```python
from build123d import *
from OCP.BRepFilletAPI import BRepFilletAPI_MakeChamfer

# Parameters (mm, degrees)
SKETCH1_W                = 40
SKETCH1_H                = 48
BOSS_EXTRUDE1_DEPTH      = 4
BOSS_EXTRUDE2_DEPTH      = 11.15
BOSS_EXTRUDE2_DEPTH_BACK = 4
SKETCH5_W                = 40
SKETCH5_H                = 4.325
SKETCH5_W_2              = 18
SKETCH5_H_2              = 5
SKETCH5_H_3              = 6
FILLET1_R                = 4
SKETCH6_R                = 1.35
CUT_EXTRUDE4_DEPTH       = 58.214705278
CHAMFER2_SIZE            = 2
SKETCH7_W                = 40
SKETCH7_H                = 6.5
CUT_EXTRUDE5_DEPTH       = 3
FILLET2_R                = 3
CHAMFER3_SIZE            = 3
CHAMFER3_SIZE2           = 1
CHAMFER4_SIZE            = 3
CHAMFER4_SIZE2           = 0.5
CUT_EXTRUDE6_DEPTH       = 10
CUT_EXTRUDE6_DEPTH_BACK  = 10
CUT_EXTRUDE8_REACH       = 66.292
SKETCH12_R               = 3
SKETCH13_R               = 1.5
CUT_EXTRUDE10_DEPTH      = 11.175
CUT_EXTRUDE7_DEPTH       = 1.25
CUT_EXTRUDE7_DEPTH_BACK  = 1.25


with BuildPart() as part:
    # Sketch1 → Boss-Extrude1 (new body)
    with BuildSketch(Plane.XY):
        with Locations((20, 14)):
            Rectangle(SKETCH1_W, SKETCH1_H)
    extrude(amount=BOSS_EXTRUDE1_DEPTH)

    # Sketch5 → Boss-Extrude2 (add, two sides: drawn at the far end of the back side and taken through both)
    with BuildSketch(Plane.XY.offset(4).offset(-BOSS_EXTRUDE2_DEPTH_BACK)):
        Polygon((1.8, 8.125), (0, 8.125), (0, 15.5), (40, 15.5), (40, 8.825), (28, 8.825), (27.1625, 10.5), (13.70350416, 10.5), (12.51600416, 8.125), (10, 8.125), (9.4, 6.925), (7.4, 6.925), (6.8, 8.125), (5, 8.125), (4.4, 6.925), (2.4, 6.925), align=None)
        with Locations((20, 3.1625)):
            Rectangle(SKETCH5_W, SKETCH5_H)
        with Locations((20, -7.5)):
            Rectangle(SKETCH5_W_2, SKETCH5_H_2)
        with Locations((20, 35)):
            Rectangle(SKETCH5_W, SKETCH5_H_3)
    extrude(amount=BOSS_EXTRUDE2_DEPTH + BOSS_EXTRUDE2_DEPTH_BACK)

    # Fillet1
    fillet1_edges = [part.edges().sort_by_distance(p)[0] for p in [
        (20, 32, 4),
        (20, 1, 4),
    ]]
    fillet(fillet1_edges, radius=FILLET1_R)

    # Sketch6 → Cut-Extrude4 (cut, through all)
    with BuildSketch(Plane.XY.offset(15.15)):
        with Locations((7.5, 35)):
            Circle(SKETCH6_R)
        with Locations((7.5, 12)):
            Circle(SKETCH6_R)
        with Locations((32.5, 35)):
            Circle(SKETCH6_R)
        with Locations((32.5, 12)):
            Circle(SKETCH6_R)
    extrude(amount=-CUT_EXTRUDE4_DEPTH, mode=Mode.SUBTRACT)

    # Chamfer2
    chamfer2_edges = [part.edges().sort_by_distance(p)[0] for p in [
        (40, 8.825, 9.575),
        (0, 15.5, 9.575),
        (40, 15.5, 9.575),
    ]]
    chamfer(chamfer2_edges, length=CHAMFER2_SIZE)

    # Sketch7 → Cut-Extrude5 (cut)
    with BuildSketch(Plane.XY.offset(4)):
        with Locations((20, 18.75)):
            Rectangle(SKETCH7_W, SKETCH7_H)
    extrude(amount=-CUT_EXTRUDE5_DEPTH, mode=Mode.SUBTRACT)

    # Fillet2
    fillet2_edges = [part.edges().sort_by_distance(p)[0] for p in [
        (20, 15.5, 1),
        (20, 22, 1),
    ]]
    fillet(fillet2_edges, radius=FILLET2_R - 0.0001)  # a hair under: the kernel refuses the full size

    # Chamfer3: one chamfer whose edges measure the first distance from different faces: ONE call of the kernel's chamfer builder (chamfer() names one face for all edges)
    chamfer3_edges_1 = [part.edges().sort_by_distance(p)[0] for p in [
        (3.4, 6.925, 15.15),
    ]]
    chamfer3_side_1 = [part.faces().sort_by_distance(p)[0] for p in [
        (3.4, 6.925, 9.575),
    ]]
    chamfer3_edges_2 = [part.edges().sort_by_distance(p)[0] for p in [
        (8.4, 6.925, 15.15),
    ]]
    chamfer3_side_2 = [part.faces().sort_by_distance(p)[0] for p in [
        (8.4, 6.925, 9.575),
    ]]
    chamfer3 = BRepFilletAPI_MakeChamfer(part.part.solid().wrapped)
    for e in chamfer3_edges_1:
        chamfer3.Add(CHAMFER3_SIZE, CHAMFER3_SIZE2, e.wrapped, chamfer3_side_1[0].wrapped)  # the first distance lies on this face
    for e in chamfer3_edges_2:
        chamfer3.Add(CHAMFER3_SIZE, CHAMFER3_SIZE2, e.wrapped, chamfer3_side_2[0].wrapped)  # the first distance lies on this face
    add(Compound.cast(chamfer3.Shape()), mode=Mode.REPLACE)

    # Chamfer4
    chamfer4_edges = [part.edges().sort_by_distance(p)[0] for p in [
        (20, 5.325, 15.15),
    ]]
    chamfer4_side = [part.faces().sort_by_distance(p)[0] for p in [
        (20, 5.325, 9.575),
    ]]
    chamfer(chamfer4_edges, length=CHAMFER4_SIZE, length2=CHAMFER4_SIZE2, reference=chamfer4_side[0])

    # Sketch8 → Cut-Extrude6 (cut, two sides: drawn at the far end of the back side and taken through both)
    with BuildSketch(Plane(origin=(20, 0, 0), x_dir=(0, 0, -1), z_dir=(1, 0, 0)).offset(-CUT_EXTRUDE6_DEPTH_BACK)):
        with BuildLine():
            Line((-9, 34.15), (-18.856272107, 34.15))
            Line((-18.856272107, 34.15), (-18.856272107, 21.85))
            Line((-18.856272107, 21.85), (-9, 21.85))
            ThreePointArc((-9, 21.85), (-2.85, 28), (-9, 34.15))
        make_face()
        with BuildLine():
            Line((-18.856272107, -10.437196649), (-18.856272107, -3.158858698))
            Line((-18.856272107, -3.158858698), (-13.348706704, 2.348706704))
            ThreePointArc((-13.348706704, 2.348706704), (-3.318140875, 0.353503109), (-9, -8.15))
            Line((-9, -8.15), (-9, -10.437196649))
            Line((-9, -10.437196649), (-18.856272107, -10.437196649))
        make_face()
    extrude(amount=CUT_EXTRUDE6_DEPTH + CUT_EXTRUDE6_DEPTH_BACK, mode=Mode.SUBTRACT)

    # Cut-Extrude8: up to this face of the body (flat: up to its plane)
    cut_extrude8_end = Plane(part.part.faces().sort_by_distance((20, 15.5, 9.574944444))[0])
    # Sketch12 → Cut-Extrude8 (cut, up to the picked face)
    with BuildSketch(Plane(origin=(0, 38, 0), x_dir=(1, 0, 0), z_dir=(0, 1, 0)), mode=Mode.PRIVATE) as cut_extrude8_sk1:
        with Locations(Location((15.4, -9, 0), (0, 0, 270))):
            Circle(SKETCH12_R)
    cut_extrude8_tool1 = split(extrude(cut_extrude8_sk1.sketch, amount=-CUT_EXTRUDE8_REACH, mode=Mode.PRIVATE), bisect_by=cut_extrude8_end, keep=Keep.BOTH, mode=Mode.PRIVATE)
    add(cut_extrude8_tool1.solids().sort_by(Axis((15.4, 38, 9), (0, -1, 0)))[0], mode=Mode.SUBTRACT)

    # Sketch13 → Cut-Extrude10 (cut)
    with BuildSketch(Plane(origin=(0, 15.5, 0), x_dir=(1, 0, 0), z_dir=(0, 1, 0))):
        with Locations(Location((15.4, -9, 0), (0, 0, 180))):
            Circle(SKETCH13_R)
    extrude(amount=-CUT_EXTRUDE10_DEPTH, mode=Mode.SUBTRACT)

    # Sketch9 → Cut-Extrude7 (cut, two sides: drawn at the far end of the back side and taken through both)
    with BuildSketch(Plane.XZ.offset(-13).offset(-CUT_EXTRUDE7_DEPTH_BACK)):
        Polygon((12.5, 16.815347994), (18.3, 16.815347994), (18.3, 7.325684219), (15.4, 5.651368439), (12.5, 7.325684219), align=None)
    extrude(amount=CUT_EXTRUDE7_DEPTH + CUT_EXTRUDE7_DEPTH_BACK, mode=Mode.SUBTRACT)


solid = part.part
```
Design review of the part built by this model. Coordinates are the model's own, in mm. A direction names the side the tool comes from. Coordinates: 2 decimals unless noted, no trailing zeros. Write each loop counter-clockwise with the first axis right and the second up, starting at its lowest first coordinate (ties: lowest second). Pieces come first, ordered by that corner, then holes. Notation, with made-up numbers: M 46.25,-11.5 L 84.25,-11.5 A24 ccw 84.25,25.5 Z; hole C 62.5,-1 d1. An arc over 180 degrees is marked long. Answer as a JSON object with one key per item and string values.
Item 1: Wall thickness on probe 1 along Y at (x, z) = (7.5, 11.5) (3 decimals); probe 2 along Y at (x, z) = (9, 11.5) (3 decimals); probe 3 along Y at (x, z) = (20, 9.25) (3 decimals): over which ranges is each line inside the solid? List them lowest first.
Outcome:
{"probe 1": "1 to 5.325, 6.925 to 10.65, 13.35 to 15.5, 32 to 33.65, 36.35 to 38", "probe 2": "1 to 5.325, 6.925 to 15.5, 32 to 38", "probe 3": "4.145 to 5.325, 10.5 to 15.5, 34.15 to 38"}
Item 2: Add section D-D, the plane y = 29. Give the boundary of the cut face in (x, z).
Outcome:
{"outline": "M 0,0 L 40,0 L 40,4.13 L 30,4.13 L 30,2.93 L 10,2.93 L 10,4.13 L 0,4.13 Z"}
Item 3: Add section A-A, the plane y = 35. Give the boundary of the cut face in (x, z), and give its area (3 significant figures).
Outcome:
{"outline": "M 0,0 L 6.15,0 L 6.15,15.15 L 0,15.15 Z; M 8.85,0 L 31.15,0 L 31.15,15.15 L 8.85,15.15 Z; M 33.85,0 L 40,0 L 40,15.15 L 33.85,15.15 Z; hole C 15.4,9 d6", "area": "496 mm²"}
Item 4: Add section B-B, the plane x = 32.5. State how many separate pieces and enclosed holes the cut face has, and give its area (3 significant figures).
Outcome:
{"separate pieces": "3", "enclosed holes": "0", "area": "290 mm²"}
Item 5: Machinability: for faces 1 (the flat face through (18.3, 13, 11)), 2 (the cylindrical face through (19.86, 0.509, 3.385)), 3 (the flat face through (3.42, 7.43, 13.67)), 4 (the flat face through (9.704, 7.533, 9.497)), which of the approach directions +Z, -Z, +X, -X, +Y, -Y give a long, thin tool a straight path to every point of the face, cutting with its end or side? Answer none if there is none.
Outcome:
{"face 1": "+Z", "face 2": "none", "face 3": "+Z, +X, -X", "face 4": "+Z, +X"}
Item 6: Draft analysis for pull direction Y (two halves, no side actions). For faces 5 (the flat face through (20, 14, 0)), 6 (the flat face through (33, 8.825, 9)), 7 (the flat face through (20, 38, 7)), state which applies: pulls with the +Y half, pulls with the -Y half, needs draft (parallel to the pull), parting line crosses it, or undercut.
Outcome:
{"face 5": "needs draft", "face 6": "undercut", "face 7": "pulls with the +Y half"}
Item 7: Insertion check: pin 1 Ø4 at (x, y) = (35, 4) entering from -Z; pin 2 Ø5 at (y, z) = (17.5, 12.5) entering from -X; pin 3 Ø0.6 at (x, z) = (8.5, 6) entering from -Y; pin 4 Ø3.5 at (x, y) = (32.5, -7.5) entering from +Z. Each pin has a flat end and moves straight along its axis. Give the tip position at first contact, or say it passes through.
Outcome:
{"pin 1": "z = 0", "pin 2": "x = 1.5", "pin 3": "y = 0.27", "pin 4": "z = 4"}
